Work out the finished part from the listing and answer in its coordinate system (mm). A direction names the side the tool comes from. Coordinates: 2 decimals unless noted, no trailing zeros. Order: outer loops, then holes, each group sorted by start corner. A loop starts at its lowest first (then second) coordinate and runs counter-clockwise, first axis right, second up. Notation, with made-up numbers: M 55,86.5 L 113,86.5 A15 ccw 113,106.5 Z; hole C 3.25,-4 d1. An arc over 180 degrees is marked long. Use a Markdown table: item, result.
from build123d import *

# Parameters (mm, degrees)
SKETCH1_R           = 5
SKETCH1_R_2         = 2.5
BOSS_EXTRUDE1_DEPTH = 5
SKETCH7_R           = 0.6
CUT_EXTRUDE1_DEPTH  = 10
SKETCH8_R           = 0.6
CUT_EXTRUDE2_DEPTH  = 2.5


with BuildPart() as part:
    # Sketch1 → Boss-Extrude1 (new body)
    with BuildSketch(Plane.XY):
        with BuildLine():
            Line((0, 7.5), (25, 7.5))
            ThreePointArc((25, 7.5), (32.5, 0), (25, -7.5))
            Line((25, -7.5), (0, -7.5))
            ThreePointArc((0, -7.5), (-7.5, 0), (0, 7.5))
        make_face()
        Circle(SKETCH1_R, mode=Mode.SUBTRACT)
        with Locations((25, 0)):
            Circle(SKETCH1_R_2, mode=Mode.SUBTRACT)
    extrude(amount=BOSS_EXTRUDE1_DEPTH)

    # Sketch7 → Cut-Extrude1 (cut)
    with BuildSketch(Plane(origin=(0, 0, 0), x_dir=(-1, 0, 0), z_dir=(0, 0, -1))):
        with Locations((-4.45, 0)):
            Circle(SKETCH7_R)
        with Locations((-6.45, 0)):
            Circle(SKETCH7_R)
        with Locations((-8.45, 0)):
            Circle(SKETCH7_R)
        with Locations((-10.45, 0)):
            Circle(SKETCH7_R)
        with Locations((-12.45, 0)):
            Circle(SKETCH7_R)
        with Locations((-14.45, 0)):
            Circle(SKETCH7_R)
    extrude(amount=-CUT_EXTRUDE1_DEPTH, mode=Mode.SUBTRACT)

    # Sketch8 → Cut-Extrude2 (cut)
    # profile 1 of 3: a face of its own
    with BuildSketch(Plane(origin=(0, 0, 0), x_dir=(-1, 0, 0), z_dir=(0, 0, -1))):
        with BuildLine():
            Line((-1.038062284, 4.891055785), (-14.865224913, 1.956422314))
            ThreePointArc((-14.865224913, 1.956422314), (-13.438479361, 1.72534808), (-12.54, 0.593211598))
            ThreePointArc((-12.54, 0.593211598), (-12.058847856, 0.454972527), (-11.85, 0))
            Line((-11.85, 0), (-11.05, 0))
            ThreePointArc((-11.05, 0), (-10.45, 0.6), (-9.85, 0))
            Line((-9.85, 0), (-9.05, 0))
            ThreePointArc((-9.05, 0), (-8.45, 0.6), (-7.85, 0))
            Line((-7.85, 0), (-7.05, 0))
            ThreePointArc((-7.05, 0), (-6.45, 0.6), (-5.85, 0))
            Line((-5.85, 0), (-5.05, 0))
            ThreePointArc((-5.05, 0), (-5.035714775, 0.130146849), (-4.993539326, 0.254096441))
            ThreePointArc((-4.993539326, 0.254096441), (-3.803998224, 3.244934131), (-1.038062284, 4.891055785))
        make_face()
    # profile 2 of 3: a face of its own
    with BuildSketch(Plane(origin=(0, 0, 0), x_dir=(-1, 0, 0), z_dir=(0, 0, -1))):
        with BuildLine():
            ThreePointArc((-12.54, 0.593211598), (-13.438479361, 1.72534808), (-14.865224913, 1.956422314))
            ThreePointArc((-14.865224913, 1.956422314), (-16.45, 0), (-14.865224913, -1.956422314))
            ThreePointArc((-14.865224913, -1.956422314), (-13.438479361, -1.72534808), (-12.54, -0.593211598))
            ThreePointArc((-12.54, -0.593211598), (-12.904972527, -0.391152144), (-13.05, 0))
            ThreePointArc((-13.05, 0), (-12.904972527, 0.391152144), (-12.54, 0.593211598))
        make_face()
        with Locations((-14.45, 0)):
            Circle(SKETCH8_R, mode=Mode.SUBTRACT)
    # profile 3 of 3: a face of its own
    with BuildSketch(Plane(origin=(0, 0, 0), x_dir=(-1, 0, 0), z_dir=(0, 0, -1))):
        with BuildLine():
            ThreePointArc((-12.54, -0.593211598), (-13.438479361, -1.72534808), (-14.865224913, -1.956422314))
            Line((-14.865224913, -1.956422314), (-1.038062284, -4.891055785))
            ThreePointArc((-1.038062284, -4.891055785), (-3.803998224, -3.244934131), (-4.993539326, -0.254096441))
            ThreePointArc((-4.993539326, -0.254096441), (-5.035714775, -0.130146849), (-5.05, 0))
            Line((-5.05, 0), (-5.85, 0))
            ThreePointArc((-5.85, 0), (-6.45, -0.6), (-7.05, 0))
            Line((-7.05, 0), (-7.85, 0))
            ThreePointArc((-7.85, 0), (-8.45, -0.6), (-9.05, 0))
            Line((-9.05, 0), (-9.85, 0))
            ThreePointArc((-9.85, 0), (-10.45, -0.6), (-11.05, 0))
            Line((-11.05, 0), (-11.85, 0))
            ThreePointArc((-11.85, 0), (-12.058847856, -0.454972527), (-12.54, -0.593211598))
        make_face()
    extrude(amount=-CUT_EXTRUDE2_DEPTH, mode=Mode.SUBTRACT)


with BuildPart() as cut_extrude2_kept_piece:
    # of the separate pieces the step leaves, the one the design keeps (cut_extrude2_pieces_kept)
    add(part.part.solids().sort_by_distance((11.85, 0, 5))[0])


solid = cut_extrude2_kept_piece.part
(1) A cutting plane is placed at B-B (z = 4.25). Determine the outline of the cut face in (x, y).
Conclusion:
| item | result |
|---|---|
| outline | M 0,-7.5 L 25,-7.5 A7.5 ccw 25,7.5 L 0,7.5 A7.5 ccw Z; hole M 4.99,-0.25 A0.6 ccw 4.99,0.25 A5 ccw long Z; hole C 6.45,0 d1.2; hole C 8.45,0 d1.2; hole C 10.45,0 d1.2; hole C 12.45,0 d1.2; hole C 14.45,0 d1.2; hole C 25,0 d5 |
(2) Determine the mould class of faces 1 (the flat face through (17, 0, 0)), 2 (the cylindrical face through (22.5, 0.1, 2.5)), 3 (the flat face through (13, -7.5, 2)) for opening direction Y: pulls with the +Y half, pulls with the -Y half, needs draft (parallel to the pull), parting line crosses it, or undercut.
Conclusion:
| item | result |
|---|---|
| face 1 | needs draft |
| face 2 | undercut |
| face 3 | pulls with the -Y half |
(3) A cutting plane is placed at D-D (y = -1.25). Determine the outline of the cut face in (x, z).
Conclusion:
| item | result |
|---|---|
| outline | M -7.4,0 L -4.84,0 L -4.84,5 L -7.4,5 Z; M 4.84,2.5 L 16.01,2.5 L 16.01,0 L 22.83,0 L 22.83,5 L 4.84,5 Z; M 27.17,0 L 32.4,0 L 32.4,5 L 27.17,5 Z |
(4) Given P1, Ø2, axis at y = 2, z = 1.5, coming from the -X side; P2, Ø2, axis at y = 3, z = 4.5, coming from the +X side; P3, Ø1, axis at x = 8.45, y = 0, coming from the +Z side; P4, Ø1.4, axis at x = 10.45, y = 0, coming from the -Z side, each flat-ended and moving along its own axis, determine where each tip first touches the part or whether it passes through.
Conclusion:
| item | result |
|---|---|
| P1 | x = -7.43 |
| P2 | x = 32.23 |
| P3 | through |
| P4 | z = 2.5 |
(5) A cutting plane is placed at A-A (y = 4). Determine the outline of the cut face in (x, z).
Conclusion:
| item | result |
|---|---|
| outline | M -6.34,0 L -3,0 L -3,5 L -6.34,5 Z; M 3,2.5 L 5.24,2.5 L 5.24,0 L 31.34,0 L 31.34,5 L 3,5 Z |
(6) Straight lines are drawn through the part: L1, parallel to Y at x = 25, z = 3.45; L2, parallel to Y at x = 10, z = 4.5; L3, parallel to X at y = 1.25, z = 0.55. For each, find the intervals that lie inside material, in ascending order.
Conclusion:
| item | result |
|---|---|
| L1 | -7.5 to -2.5, 2.5 to 7.5 |
| L2 | -7.5 to -0.4, 0.4 to 7.5 |
| L3 | -7.4 to -4.84, 16.01 to 22.83, 27.17 to 32.4 |
(7) A cutting plane is placed at C-C (x = 10.45). Determine the outline of the cut face in (y, z), then the cut area to 3 significant figures.
Conclusion:
| item | result |
|---|---|
| outline | M -7.5,0 L -2.89,0 L -2.89,2.5 L -0.6,2.5 L -0.6,5 L -7.5,5 Z; M 0.6,2.5 L 2.89,2.5 L 2.89,0 L 7.5,0 L 7.5,5 L 0.6,5 Z |
| area | 57.5 mm2 |
(8) Which of the six approach directions +Z, -Z, +X, -X, +Y, -Y give full straight-line access (tool end or side, diameter ignored) to faces 4 (the cylindrical face through (9.896, -0.23, 3.732)), 5 (the cylindrical face through (16.45, 0.04, 1.23))?
Conclusion:
| item | result |
|---|---|
| face 4 | +Z, -Z |
| face 5 | -Z |
